from build123d import *

# Parameters (mm, degrees)
BOSS_EXTRUDE1_DEPTH = 15
CUT_EXTRUDE1_DEPTH  = 143.214626533
CUT_EXTRUDE3_START  = -4
CUT_EXTRUDE3_DEPTH  = 139.214626533
FILLET1_R           = 1
FILLET2_R           = 0.5
SKETCH4_W           = 15
SKETCH4_H           = 28
BOSS_EXTRUDE2_DEPTH = 7
CHAMFER1_SIZE       = 3
FILLET3_R           = 5


with BuildPart() as part:
    # Sketch1 → Boss-Extrude1 (new body)
    with BuildSketch(Plane(origin=(0, 0, 0), x_dir=(1, 0, 0), z_dir=(0, 1, 0))):
        with BuildLine():
            Line((-57.286267839, -105.443271559), (-68, -124))
            Line((-68, -124), (68, -124))
            Line((68, -124), (57.286267839, -105.443271559))
            ThreePointArc((57.286267839, -105.443271559), (0, -120), (-57.286267839, -105.443271559))
        make_face()
    extrude(amount=BOSS_EXTRUDE1_DEPTH)

    # Sketch2 → Cut-Extrude1 (cut, through all)
    with BuildSketch(Plane(origin=(0, 15, 0), x_dir=(1, 0, 0), z_dir=(0, 1, 0))):
        with BuildLine():
            Line((-52.804159001, -115.380031326), (-55.129159001, -119.407049454))
            ThreePointArc((-55.129159001, -119.407049454), (-58.441770605, -120.294661058), (-59.32938221, -116.982049454))
            Line((-59.32938221, -116.982049454), (-57.00438221, -112.955031326))
            ThreePointArc((-57.00438221, -112.955031326), (-53.691770605, -112.067419722), (-52.804159001, -115.380031326))
        make_face()
        with BuildLine():
            Line((52.804159001, -115.380031326), (55.129159001, -119.407049454))
            ThreePointArc((55.129159001, -119.407049454), (58.441770605, -120.294661058), (59.32938221, -116.982049454))
            Line((59.32938221, -116.982049454), (57.00438221, -112.955031326))
            ThreePointArc((57.00438221, -112.955031326), (53.691770605, -112.067419722), (52.804159001, -115.380031326))
        make_face()
    extrude(amount=-CUT_EXTRUDE1_DEPTH, mode=Mode.SUBTRACT)

    # Sketch3 → Cut-Extrude3 (cut, through all)
    with BuildSketch(Plane(origin=(0, 15, 0), x_dir=(1, 0, 0), z_dir=(0, 1, 0)).offset(CUT_EXTRUDE3_START)):
        with BuildLine():
            Line((-51.019656288, -116.439181962), (-53.319656288, -120.422898819))
            ThreePointArc((-53.319656288, -120.422898819), (-59.466770605, -122.070013136), (-61.113884922, -115.922898819))
            Line((-61.113884922, -115.922898819), (-58.813884922, -111.939181962))
            ThreePointArc((-58.813884922, -111.939181962), (-52.666770605, -110.292067644), (-51.019656288, -116.439181962))
        make_face()
        with BuildLine():
            Line((51.019656288, -116.439181962), (53.319656288, -120.422898819))
            ThreePointArc((53.319656288, -120.422898819), (59.466770605, -122.070013136), (61.113884922, -115.922898819))
            Line((61.113884922, -115.922898819), (58.813884922, -111.939181962))
            ThreePointArc((58.813884922, -111.939181962), (52.666770605, -110.292067644), (51.019656288, -116.439181962))
        make_face()
    extrude(amount=-CUT_EXTRUDE3_DEPTH, mode=Mode.SUBTRACT)

    # Fillet1
    fillet1_edges = [part.edges().sort_by_distance(p)[0] for p in [
        (57.286267839, 7.5, 105.443271559),
        (68, 7.5, 124),
        (-68, 7.5, 124),
        (-57.286267839, 7.5, 105.443271559),
    ]]
    fillet(fillet1_edges, radius=FILLET1_R)

    # Fillet2
    fillet2_edges = [part.edges().sort_by_distance(p)[0] for p in [
        (-58.16688221, 11, 114.96854039),
        (53.966659001, 11, 117.39354039),
        (-52.666770605, 11, 110.292067644),
        (-59.963884922, 11, 113.93104039),
        (-59.466770605, 11, 122.070013136),
        (-52.169656288, 11, 118.43104039),
        (-53.691770605, 11, 112.067419722),
        (-53.966659001, 11, 117.39354039),
        (-58.441770605, 11, 120.294661058),
        (52.666770605, 11, 110.292067644),
        (52.169656288, 11, 118.43104039),
        (59.466770605, 11, 122.070013136),
        (59.963884922, 11, 113.93104039),
        (58.16688221, 11, 114.96854039),
        (53.691770605, 11, 112.067419722),
        (58.441770605, 11, 120.294661058),
    ]]
    fillet(fillet2_edges, radius=FILLET2_R)

    # Sketch4 → Boss-Extrude2 (add)
    with BuildSketch(Plane(origin=(0, 15, 0), x_dir=(1, 0, 0), z_dir=(0, 1, 0))):
        with Locations((0, -110)):
            Rectangle(SKETCH4_W, SKETCH4_H)
    extrude(amount=-BOSS_EXTRUDE2_DEPTH)

    # Chamfer1
    # the kernel refuses this chamfer: 3, 2.828734379 mm, written as the material it adds along each edge
    with BuildSketch(Plane(origin=(-7.5, 15, 119.76539567), x_dir=(0, 0, -1), z_dir=(0, -1, 0))) as chamfer1_piece_1:
        with BuildLine():
            Line((CHAMFER1_SIZE, 0), (0.207600012, -2.792399988))
            ThreePointArc((0.207600012, -2.792399988), (0.098564019, -1.43584929), (0, 0))
            Line((0, 0), (CHAMFER1_SIZE, 0))
        make_face()
    extrude(amount=7)
    with BuildSketch(Plane(origin=(7.5, 15, 119.76539567), x_dir=(0, 0, -1), z_dir=(0, -1, 0))) as chamfer1_piece_2:
        with BuildLine():
            Line((CHAMFER1_SIZE, 0), (0.207600012, 2.792399988))
            ThreePointArc((0.207600012, 2.792399988), (0.098564019, 1.43584929), (0, 0))
            Line((0, 0), (CHAMFER1_SIZE, 0))
        make_face()
    extrude(amount=7)

    # Fillet3
    fillet3_edges = [part.edges().sort_by_distance(p)[0] for p in [
        (7.5, 11.5, 96),
        (-7.5, 11.5, 96),
    ]]
    fillet(fillet3_edges, radius=FILLET3_R)


solid = part.part
Design review of the part built by this model. Coordinates are the model's own, in mm. A direction names the side the tool comes from. Give positions to 0.01 mm unless a question says otherwise; leave off trailing zeros. Write each loop counter-clockwise with the first axis right and the second up, starting at its lowest first coordinate (ties: lowest second). Pieces come first, ordered by that corner, then holes. Notation, with made-up numbers: M 32.25,50 L 65.25,50 A7 cw 65.25,58 Z; hole C 26,9 d5. An arc over 180 degrees is marked long. Return JSON: item names as keys, results as strings. Group by question number.
Item 1: Take a section at A-A (y = 13.75). Count the separate pieces of the cut face and the enclosed holes in it, plus the area to 3 significant figures.
Item 2: Wall thickness on line 1 along X through (y, z) = (10.75, 120.75); line 2 along X through (y, z) = (10.25, 108.5); line 3 along Z through (x, y) = (47.5, 9.25): over which ranges is each line inside the solid? List them lowest first.
Item 3: Take a section at B-B (z = 107.5). Give the boundary of the cut face in (x, y), plus the area to 3 significant figures.
Item 4: The part is to be moulded in two halves that separate along X. For faces 5 (the flat face through (-1, 0, 121)), 6 (the cylindrical face through (-6, 11.45, 97.43)), 7 (the cylindrical face through (-58.274, 11.15, 114.869)), say which applies: pulls with the +X half, pulls with the -X half, needs draft (parallel to the pull), parting line crosses it, or undercut.
Item 5: Clearance check with flat-ended pins moving along their axes: pin 1 Ø1 at (x, z) = (-6.5, 109) entering from -Y; pin 2 Ø3.5 at (y, z) = (12, 106.5) entering from -X; pin 3 Ø3 at (y, z) = (10.5, 100) entering from +X; pin 4 Ø3 at (x, z) = (-54.5, 113.5) entering from -Y. State where each tip first meets the part, or that it passes through.
Item 6: Take a section at D-D (x = 5). Give the boundary of the cut face in (y, z).
Item 7: Tool access review of faces 1 (the flat face through (-1, 8, 124)), 2 (the flat face through (-7.5, 12, 109)), 3 (the flat face through (0, 8, 108)), 4 (the flat face through (52.15, 5.32, 118.4)): name each direction out of +Z, -Z, +X, -X, +Y, -Y from which nothing blocks a thin tool from reaching the whole face with its end or side.
Item 8: Take a section at C-C (y = 5.75). Give the boundary of the cut face in (x, z), plus the area to 3 significant figures.
Return value:
{
 "1": {"separate pieces": "1", "enclosed holes": "2", "area": "1,470 mm2"},
 "2": {"line 1": "x = -66.12 to -60.82, -53.61 to 53.61, 60.82 to 66.12", "line 2": "x = -59.05 to -51.26, -7.5 to 7.5, 51.26 to 59.05", "line 3": "z = 110.2 to 124"},
 "3": {"outline": "M -58.47,0 L -53.33,0 L -53.33,15 L -58.47,15 Z; M -7.5,8 L 7.5,8 L 7.5,15 L -7.5,15 Z; M 53.33,0 L 58.47,0 L 58.47,15 L 53.33,15 Z", "area": "259 mm2"},
 "4": {"face 5": "needs draft", "face 6": "pulls with the -X half", "face 7": "undercut"},
 "5": {"pin 1": "stops at y = 8", "pin 2": "stops at x = -58.91", "pin 3": "stops at x = 7.5", "pin 4": "passes through"},
 "6": {"outline": "M 0,119.9 L 8,119.9 L 8,96.67 L 15,96.67 L 15,124 L 0,124 Z"},
 "7": {"face 1": "+Z, +X, -X, +Y, -Y", "face 2": "-Z, +Y, -Y", "face 3": "-Z, -Y", "face 4": "-Y"},
 "8": {"outline": "M -67.13,122.5 L -57.77,106.28 A1 ccw -56.44,105.9 A120 cw 56.44,105.9 A1 ccw 57.77,106.28 L 67.13,122.5 A1 ccw 66.27,124 L -66.27,124 A1 ccw Z; hole M -61.11,115.92 L -58.81,111.94 A4.5 ccw -51.02,116.44 L -53.32,120.42 A4.5 ccw Z; hole M 51.02,116.44 A4.5 ccw 58.81,111.94 L 61.11,115.92 A4.5 ccw 53.32,120.42 Z", "area": "987 mm2"}
}
